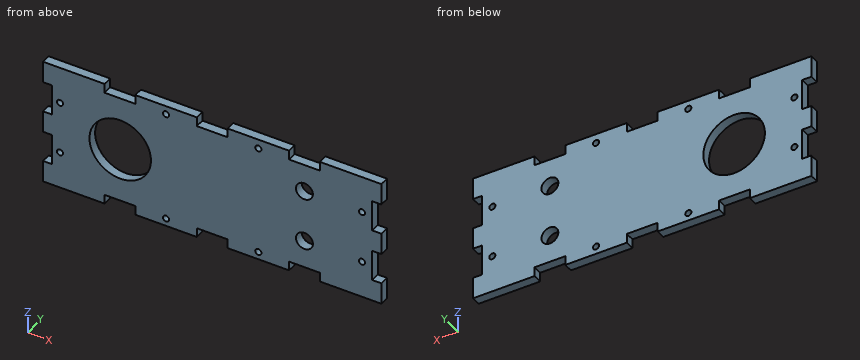
```python
from build123d import *

# Parameters (mm, degrees)
F0_R     = 1
F0_R_2   = 10
F0_R_3   = 2.75
F1_DEPTH = 3


with BuildPart() as f1:
    # F0 (on Front) → F1 (new body)
    with BuildSketch(Plane.XZ):
        Polygon((-51.975646, 2.591607), (-54.975646, 2.591607), (-54.975646, -0.908393), (-54.975646, -4.408393), (-51.975646, -4.408393), (-51.975646, -14.408393), (-54.975646, -14.408393), (-54.975646, -21.408393), (-34.975646, -21.408393), (-34.975646, -18.408393), (-24.975646, -18.408393), (-24.975646, -21.408393), (-4.975646, -21.408393), (-4.975646, -18.408393), (0.024354, -18.408393), (5.024354, -18.408393), (5.024354, -21.408393), (25.024354, -21.408393), (25.024354, -18.408393), (35.024354, -18.408393), (35.024354, -21.408393), (55.024354, -21.408393), (55.024354, -14.408393), (52.024354, -14.408393), (52.024354, -4.408393), (55.024354, -4.408393), (55.024354, -0.908393), (55.024354, 2.591607), (52.024354, 2.591607), (52.024354, 12.591607), (55.024354, 12.591607), (55.024354, 19.591607), (35.024354, 19.591607), (35.024354, 16.591607), (25.024354, 16.591607), (25.024354, 19.591607), (5.024354, 19.591607), (5.024354, 16.591607), (0.024354, 16.591607), (-4.975646, 16.591607), (-4.975646, 19.591607), (-24.975646, 19.591607), (-24.975646, 16.591607), (-34.975646, 16.591607), (-34.975646, 19.591607), (-54.975646, 19.591607), (-54.975646, 12.591607), (-51.975646, 12.591607), align=None)
        with Locations((-14.975646, -18.908393)):
            Circle(F0_R, mode=Mode.SUBTRACT)
        with Locations((-49.452938, -9.408393)):
            Circle(F0_R, mode=Mode.SUBTRACT)
        with Locations((-29.869903, -0.908393)):
            Circle(F0_R_2, mode=Mode.SUBTRACT)
        with Locations((15.024354, -18.908393)):
            Circle(F0_R, mode=Mode.SUBTRACT)
        with Locations((30.024354, -9.408393)):
            Circle(F0_R_3, mode=Mode.SUBTRACT)
        with Locations((48.734484, -9.408393)):
            Circle(F0_R, mode=Mode.SUBTRACT)
        with Locations((-49.452938, 7.591607)):
            Circle(F0_R, mode=Mode.SUBTRACT)
        with Locations((-14.975646, 16.840009)):
            Circle(F0_R, mode=Mode.SUBTRACT)
        with Locations((30.024354, 7.591607)):
            Circle(F0_R_3, mode=Mode.SUBTRACT)
        with Locations((48.734484, 7.591607)):
            Circle(F0_R, mode=Mode.SUBTRACT)
        with Locations((15.024354, 16.571959)):
            Circle(F0_R, mode=Mode.SUBTRACT)
    extrude(amount=F1_DEPTH)


solid = f1.part
```
Geometry check sheet. Reference: the model listing, model coordinates, mm. Give positions to 0.01 mm unless a question says otherwise; leave off trailing zeros. Order: outer loops, then holes, each group sorted by start corner. A loop starts at its lowest first (then second) coordinate and runs counter-clockwise, first axis right, second up. Notation, with made-up numbers: (42.25, 79.5) - (94.25, 79.5) arc R17 cw to (94.25, 101.5) - close; hole circle Ø4 at (-32, 71). An arc over 180 degrees is marked (long way). Answer in a Markdown table with one row per item. Add a question column.
Q1. Cross-section at D-D, the plane y = -1.5. Count the separate pieces of the cut face and the enclosed holes in it, then the cut area to 3 significant figures.
Q2. Cross-section at A-A, the plane x = -34. Enter the section's corners in (y, z), then the cut area to 3 significant figures.
Q3. Cross-section at C-C, the plane x = 0. Enter the section's corners in (y, z), then the cut area to 3 significant figures.
Q4. Cross-section at B-B, the plane z = 1.5. Enter the section's corners in (x, y).
Q5. Material ranges on probe 1 along X at (y, z) = (-0.5, 18); probe 2 along X at (y, z) = (-2.8, -18.5); probe 3 along Z at (x, y) = (0, -0.75), recorded low to high. Write a range as from..to.
Q6. Gauge pin test, flat ends, axial feed: pin 1 (1.5 mm diameter, centred on y = -1, z = 6.5, fed in from -X); pin 2 (1.6 mm diameter, centred on x = 15.02, z = 16.57, fed in from +Y); pin 3 (0.9 mm diameter, centred on y = -1.5, z = -7.5, fed in from +X). Record the tip position at first contact, or that the pin passes through.
Check values:
| question | item | result |
|---|---|---|
| 1 | separate pieces | 1 |
| 1 | enclosed holes | 11 |
| 1 | area | 3,820 mm^2 |
| 2 | outline | (-3, -18.41) - (0, -18.41) - (0, -10.02) - (-3, -10.02) - close; (-3, 8.2) - (0, 8.2) - (0, 16.59) - (-3, 16.59) - close |
| 2 | area | 50.4 mm^2 |
| 3 | outline | (-3, -18.41) - (0, -18.41) - (0, 16.59) - (-3, 16.59) - close |
| 3 | area | 105 mm^2 |
| 4 | outline | (-54.98, -3) - (-39.58, -3) - (-39.58, 0) - (-54.98, 0) - close; (-20.16, -3) - (55.02, -3) - (55.02, 0) - (-20.16, 0) - close |
| 5 | probe 1 | x = -54.98..-34.98, -24.98..-4.98, 5.02..25.02, 35.02..55.02 |
| 5 | probe 2 | x = -54.98..-34.98, -24.98..-15.89, -14.06..-4.98, 5.02..14.11, 15.94..25.02, 35.02..55.02 |
| 5 | probe 3 | z = -18.41..16.59 |
| 6 | pin 1 | stops at x = -51.98 |
| 6 | pin 2 | passes through |
| 6 | pin 3 | stops at x = 52.02 |
